Could you check a few things on this model? Use its own coordinates, in mm. A direction names the side the tool comes from. Round coordinates to 2 decimals unless told otherwise and drop trailing zeros. Order: outer loops, then holes, each group sorted by start corner. A loop starts at its lowest first (then second) coordinate and runs counter-clockwise, first axis right, second up. Notation, with made-up numbers: (56.5, 34) -> (80.5, 34) arc R27 ccw to (80.5, 53) -> close; hole circle Ø7 at (78.5, 67). An arc over 180 degrees is marked (long way). Put each result on its own line as item: value. Start each with the question number.
from build123d import *

# Parameters (mm, degrees)
SKETCH1_R                  = 2.4892
BOSS_EXTRUDE1_DEPTH        = 3.175
SKETCHED_START             = -52
SKETCHED_BEND2_DEPTH       = 52
SKETCHED_START_2           = -25.4
SKETCHED_BEND2_2_DEPTH     = 12.7
SKETCHED_START_3           = -41.835294118
SKETCHED_BEND2_3_OUTLINE_W = 3.175
SKETCHED_BEND2_3_OUTLINE_H = 12.7
SKETCHED_BEND2_3_DEPTH     = 16.435294118
SKETCHED_BEND2_4_DEPTH     = 20.459192
SKETCHED_START_4           = -50.8
SKETCHED_BEND2_5_OUTLINE_W = 3.175
SKETCHED_BEND2_5_OUTLINE_H = 12.7
SKETCHED_BEND2_5_DEPTH     = 48.117252
SKETCHED_START_5           = -4.940808
SKETCHED_BEND2_6_DEPTH     = 4.940808
SKETCHED_START_6           = -3.175
SKETCHED_BEND2_7_DEPTH     = 3.175
SKETCH13_R                 = 1.1303
CUT_EXTRUDE2_DEPTH         = 71.302458254
FILLET1_R                  = 3.175
SKETCH14_W                 = 22.407113123
SKETCH14_H                 = 6.985
CUT_EXTRUDE3_DEPTH         = 69.199553227
FILLET2_R                  = 3.175


with BuildPart() as part:
    # Sketch1 → Boss-Extrude1 (new body)
    # profile 1 of 2: a face of its own
    with BuildSketch(Plane(origin=(0, 0, 0), x_dir=(1, 0, 0), z_dir=(0, 1, 0))):
        Polygon((6.35, 0), (25.4, 0), (34.925, 0), (34.925, 25.4), (26.986065751, 25.4), (10.476065751, 25.4), (6.35, 25.4), align=None)
        with Locations(Location((22.225, 6.35, 0), (0, 0, 270))):
            Circle(SKETCH1_R, mode=Mode.SUBTRACT)
        with Locations(Location((22.225, 19.05, 0), (0, 0, 270))):
            Circle(SKETCH1_R, mode=Mode.SUBTRACT)
    # profile 2 of 2: a face of its own
    with BuildSketch(Plane(origin=(0, 0, 0), x_dir=(1, 0, 0), z_dir=(0, 1, 0))):
        Polygon((-12.7, 0), (6.35, 0), (6.35, 25.4), (0, 25.4), (-19.05, 25.4), (-19.05, 41.835294118), (-23.415467049, 44.91680027), (-31.75, 50.8), (-31.75, 12.7), (-23.415467049, 7.143644699), align=None)
    extrude(amount=BOSS_EXTRUDE1_DEPTH)

    # Sketched Bend2: read off the stored shape, not the designer's step
    # Sketched Bend2 outline → Sketched Bend2 (cut)
    with BuildSketch(Plane.XY.offset(SKETCHED_START)):
        with BuildLine():
            ThreePointArc((3.175, 0), (-1e-09, 0.850738686), (-2.324261315, 3.175))
            Line((-2.324261315, 3.175), (-31.75, 3.175))
            Line((-31.75, 3.175), (-31.75, 0))
            Line((-31.75, 0), (3.175, 0))
        make_face()
    extrude(amount=SKETCHED_BEND2_DEPTH, mode=Mode.SUBTRACT)

    # Sketched Bend2 2 outline → Sketched Bend2 2 (add)
    with BuildSketch(Plane.XY.offset(SKETCHED_START_2)):
        with BuildLine():
            ThreePointArc((3.175, 3.175), (0.92993597, 4.10493597), (0, 6.35))
            Line((0, 6.35), (0, 33.794082494))
            Line((0, 33.794082494), (-3.175, 33.794082494))
            Line((-3.175, 33.794082494), (-3.175, 6.35))
            ThreePointArc((-3.175, 6.35), (-2.958628997, 4.706499064), (-2.324261315, 3.175))
            Line((-2.324261315, 3.175), (3.175, 3.175))
        make_face()
    extrude(amount=SKETCHED_BEND2_2_DEPTH)

    # Sketched Bend2 3 outline → Sketched Bend2 3 (add)
    with BuildSketch(Plane.XY.offset(SKETCHED_START_3)):
        with Locations((-1.5875, 27.444082494)):
            Rectangle(SKETCHED_BEND2_3_OUTLINE_W, SKETCHED_BEND2_3_OUTLINE_H)
    extrude(amount=SKETCHED_BEND2_3_DEPTH)

    # Sketched Bend2 4 outline → Sketched Bend2 4 (add)
    with BuildSketch(Plane.XY.offset(SKETCHED_START_2)):
        with BuildLine():
            ThreePointArc((3.175, 3.175), (0.92993597, 4.10493597), (0, 6.35))
            Line((0, 6.35), (0, 21.094082494))
            Line((0, 21.094082494), (-3.175, 21.094082494))
            Line((-3.175, 21.094082494), (-3.175, 6.35))
            ThreePointArc((-3.175, 6.35), (-2.958628997, 4.706499064), (-2.324261315, 3.175))
            Line((-2.324261315, 3.175), (3.175, 3.175))
        make_face()
    extrude(amount=SKETCHED_BEND2_4_DEPTH)

    # Sketched Bend2 5 outline → Sketched Bend2 5 (add)
    with BuildSketch(Plane.XY.offset(SKETCHED_START_4)):
        with Locations((-1.5875, 27.444082494)):
            Rectangle(SKETCHED_BEND2_5_OUTLINE_W, SKETCHED_BEND2_5_OUTLINE_H)
    extrude(amount=SKETCHED_BEND2_5_DEPTH)

    # Sketched Bend2 6 outline → Sketched Bend2 6 (add)
    with BuildSketch(Plane.XY.offset(SKETCHED_START_5)):
        with BuildLine():
            ThreePointArc((3.175, 3.175), (0.92993597, 4.10493597), (0, 6.35))
            Line((0, 6.35), (0, 21.094082494))
            Line((0, 21.094082494), (-3.175, 21.094082494))
            Line((-3.175, 21.094082494), (-3.175, 6.35))
            ThreePointArc((-3.175, 6.35), (-2.958628997, 4.706499064), (-2.324261315, 3.175))
            Line((-2.324261315, 3.175), (3.175, 3.175))
        make_face()
    extrude(amount=SKETCHED_BEND2_6_DEPTH)

    # Sketched Bend2 7 outline → Sketched Bend2 7 (cut)
    with BuildSketch(Plane.YZ.offset(SKETCHED_START_6)):
        Polygon((21.094082494, 0), (14.744082494, 0), (33.794082494, -12.7), (33.794082494, -2.682748), (21.094082494, -2.682748), align=None)
        Polygon((21.094082494, -50.8), (33.794082494, -50.8), (21.094082494, -41.835294118), align=None)
    extrude(amount=SKETCHED_BEND2_7_DEPTH, mode=Mode.SUBTRACT)

    # Sketch13 → Cut-Extrude2 (cut, through all)
    with BuildSketch(Plane(origin=(0, 0, 0), x_dir=(0, 0, -1), z_dir=(1, 0, 0))):
        with Locations(Location((42.418, 28.575, 0), (0, 0, 90))):
            Circle(SKETCH13_R)
        with Locations(Location((36.068, 28.575, 0), (0, 0, 90))):
            Circle(SKETCH13_R)
        with Locations(Location((29.718, 28.575, 0), (0, 0, 90))):
            Circle(SKETCH13_R)
        with Locations(Location((23.368, 28.575, 0), (0, 0, 90))):
            Circle(SKETCH13_R)
        with Locations(Location((17.018, 28.575, 0), (0, 0, 90))):
            Circle(SKETCH13_R)
    extrude(amount=-CUT_EXTRUDE2_DEPTH, mode=Mode.SUBTRACT)

    # Fillet1
    fillet1_edges = [part.edges().sort_by_distance(p)[0] for p in [
        (-1.5875, 21.094082494, -41.835294118),
        (-1.5875, 21.094082494, -25.4),
        (-1.5875, 14.744082494, 0),
        (-1.5875, 33.794082494, -12.7),
        (-1.5875, 33.794082494, -50.8),
        (34.925, 1.5875, -25.4),
        (34.925, 1.5875, 0),
    ]]
    fillet(fillet1_edges, radius=FILLET1_R)

    # Sketch14 → Cut-Extrude3 (cut, through all)
    with BuildSketch(Plane(origin=(0, 0, 0), x_dir=(0, 0, -1), z_dir=(1, 0, 0))):
        with Locations((36.603556561, 21.411582494)):
            Rectangle(SKETCH14_W, SKETCH14_H)
    extrude(amount=-CUT_EXTRUDE3_DEPTH, mode=Mode.SUBTRACT)

    # Fillet2
    fillet2_edges = [part.edges().sort_by_distance(p)[0] for p in [
        (-1.5875, 24.904082494, -44.524705882),
        (-1.5875, 24.904082494, -25.4),
    ]]
    fillet(fillet2_edges, radius=FILLET2_R)


solid = part.part
1. Which directions (+Z, -Z, +X, -X, +Y, -Y) give clear straight access to the entire face, cutting with the end or side of a thin tool? Please do faces 1 (the face through (-2, 24.904, -36)), 2 (the face through (0, 20, -19)), 3 (the face through (-1.57, 29.1, -37.07)).
2. I need wall thicknesses on L1, parallel to X at y = 27.5, z = -18 (3 decimals); L2, parallel to Y at x = 23, z = -24 (3 decimals); L3, parallel to X at y = 2, z = -6 (3 decimals). Which ranges of each line are inside material? Lowest first, please.
3. If we section it at D-D, the plane y = 12.5: Please give me the cut outline in (x, z) (3 decimals), then the cut area to 3 significant figures.
4. For pin 1 Ø13.5 at (y, z) = (19.5, -35.5) entering from +X; pin 2 Ø3.5 at (x, z) = (-1, -35.5) entering from -Y; pin 3 Ø11 at (x, y) = (7, 7.5) entering from -Z, each with a flat end and sliding along its axis, tell me the tip position at first contact or that it passes through.
5. If we section it at A-A, the plane z = -19.05: Please give me the cut outline in (x, y) (3 decimals), then the cut area to 3 significant figures.
6. If we section it at B-B, the plane x = 23: Please give me the cut outline in (y, z) (3 decimals).
7. If we section it at C-C, the plane x = 15: Please give me the cut outline in (y, z) (3 decimals), then the cut area to 3 significant figures.
8. Thinking about a two-plate mould opening in Z: for faces 4 (the face through (19.795, 1.565, -6.89)), 5 (the face through (-1.565, 14.69, -0.132)), 6 (the face through (-2, 33.794, -30)), which applies, +Z half, -Z half, draft (parallel to the pull), parting line (faces both ways), or undercut?
Results below:
1. face 1: -Z, +X, -X, -Y
1. face 2: +Z, -Z, +X, +Y
1. face 3: +X, -X
2. L1: -3.175 to 0
2. L2: 0 to 3.175
2. L3: -1.451 to 19.761, 24.689 to 34.925
3. outline: (-3.175, -25.4) -> (0, -25.4) -> (0, 0) -> (-3.175, 0) -> close
3. area: 80.6 mm2
4. pin 1: x = 0
4. pin 2: y = 24.9
4. pin 3: z = -25.4
5. outline: (-3.175, 6.35) arc R6.35 ccw to (3.175, 0) -> (19.736, 0) -> (19.736, 3.175) -> (3.175, 3.175) arc R3.175 cw to (0, 6.35) -> (0, 33.794) -> (-3.175, 33.794) -> close; (24.714, 0) -> (34.925, 0) -> (34.925, 3.175) -> (24.714, 3.175) -> close
5. area: 196 mm2
6. outline: (0, -25.4) -> (3.175, -25.4) -> (3.175, -21.415) -> (0, -21.415) -> close; (0, -16.685) -> (3.175, -16.685) -> (3.175, -8.715) -> (0, -8.715) -> close; (0, -3.985) -> (3.175, -3.985) -> (3.175, 0) -> (0, 0) -> close
7. outline: (0, -25.4) -> (3.175, -25.4) -> (3.175, 0) -> (0, 0) -> close
7. area: 80.6 mm2
8. face 4: undercut
8. face 5: +Z half
8. face 6: draft
